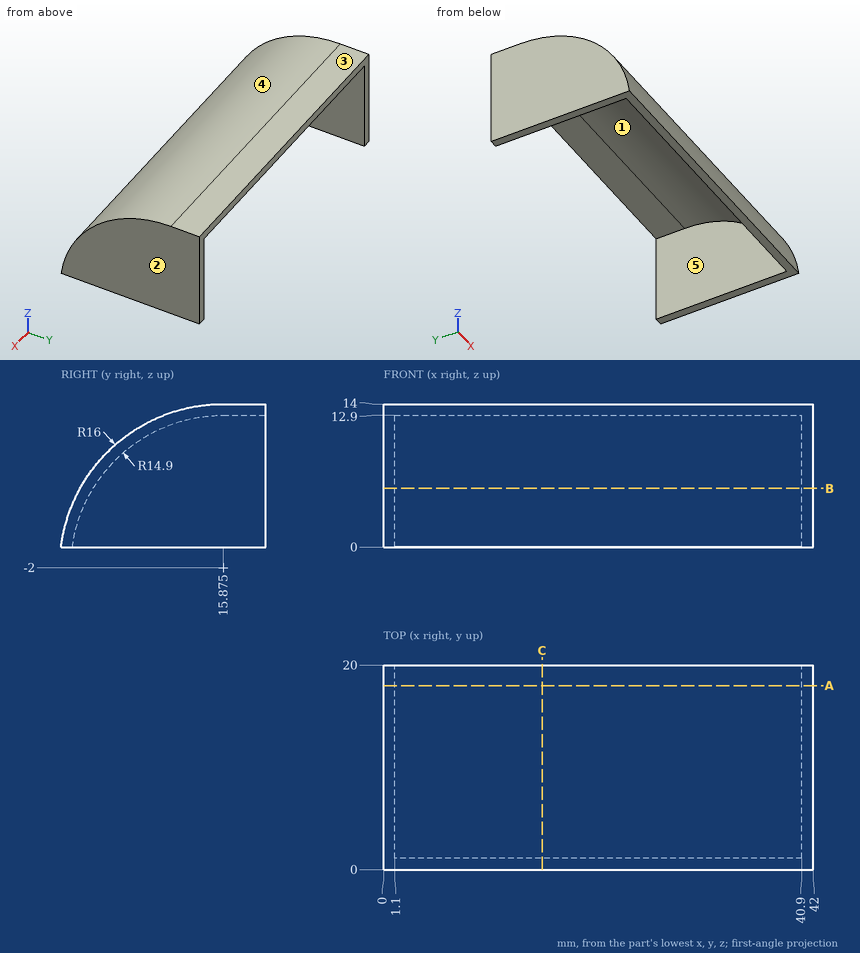
Study the drawing (mm; zero at the part's minimum x, y, z) and answer. A direction names the side the tool comes from. Round coordinates to 2 decimals unless told otherwise and drop trailing zeros. Write each loop counter-clockwise with the first axis right and the second up, starting at its lowest first coordinate (ties: lowest second). Pieces come first, ordered by that corner, then holes.
1) Flat-ended cylindrical pins translate along their axes: P1, Ø4, axis at x = 35.5, y = 5, coming from the +Z side; P2, Ø3.5, axis at x = 21.5, y = 19, coming from the -Z side; P3, Ø12, axis at x = 12, y = 12.5, coming from the -Z side. Find the tip coordinate at first contact, or state that the pin passes through.
2) Which of the six approach directions +Z, -Z, +X, -X, +Y, -Y give full straight-line access (tool end or side, diameter ignored) to the marked faces 4 and 5?
3) Determine the mould class of the marked faces 1, 2 and 3 for opening direction X: pulls with the +X half, pulls with the -X half, needs draft (parallel to the pull), parting line crosses it, or undercut.
4) A cutting plane is placed at C-C on x = 15.5. Determine the outline of the cut face in (y, z) (1 decimal).
5) A cutting plane is placed at A-A on y = 18. Determine the outline of the cut face in (x, z).
6) Consider probe 1 along X at (y, z) = (3.75, 5); probe 2 along Z at (x, y) = (10, 17.75); probe 3 along Y at (x, z) = (22.5, 6.5) (1 decimal). Determine where each line is inside the solid, lowest interval first.
7) A cutting plane is placed at B-B on z = 5.75. Determine the outline of the cut face in (x, y).
Entries:
1. P1: stops at z = 11.31
1. P2: stops at z = 12.9
1. P3: stops at z = 9.58
2. face 4: +Z, +X, -X, -Y
2. face 5: -Z, +Y
3. face 1: undercut
3. face 2: pulls with the +X half
3. face 3: needs draft
4. outline: (0, 0) - (1.1, 0) arc R14.9 cw to (15.9, 12.9) - (20, 12.9) - (20, 14) - (15.9, 14) arc R16 ccw to start
5. outline: (0, 0) - (1.1, 0) - (1.1, 12.9) - (40.9, 12.9) - (40.9, 0) - (42, 0) - (42, 14) - (0, 14) - close
6. probe 1: x = 0 to 1.1, 40.9 to 42
6. probe 2: z = 12.9 to 14
6. probe 3: y = 2.3 to 3.6
7. outline: (0, 1.88) - (42, 1.88) - (42, 20) - (40.9, 20) - (40.9, 3.15) - (1.1, 3.15) - (1.1, 20) - (0, 20) - close
